The listing builds one solid part. Answer for the finished solid, in the listing's coordinates (mm). A direction names the side the tool comes from. Round coordinates to 2 decimals unless told otherwise and drop trailing zeros. Order: outer loops, then holes, each group sorted by start corner. A loop starts at its lowest first (then second) coordinate and runs counter-clockwise, first axis right, second up. Notation, with made-up numbers: M 30.25,1 L 73.25,1 A13 cw 73.25,16 Z; hole C 62,-29.75 d1. An arc over 180 degrees is marked long. Write item = value, one per line. Start each with the question number.
(1) A cutting plane is placed at A-A, the plane y = 9.5. Determine the outline of the cut face in (x, z).
(2) For a pull along X with two mould halves and no side action, classify faces 1 (the face through (-27.5, 2, 32)), 2 (the face through (-7.615, 1.462, 32.255)), 3 (the face through (-2, 7, 50)), 4 (the face through (-9, 2, 58)) as released by +X, released by -X, zero draft, split by the parting line, or undercut.
(3) Each of these flat-tipped pins is pushed along its axis until it touches: pin 1 (10 mm diameter, centred on y = 7.5, z = 38.5, fed in from +X); pin 2 (6 mm diameter, centred on x = -20, z = 42, fed in from +Y); pin 3 (5 mm diameter, centred on y = 2.5, z = 56, fed in from +X); pin 4 (3 mm diameter, centred on x = -5, z = 44, fed in from +Y). Where does it stop, or does it pass through?
(4) A cutting plane is placed at C-C, the plane z = 8.5. Determine the outline of the cut face in (x, y), and give its area (3 significant figures).
(5) Straight lines are drawn through the part: probe 1 along Y at (x, z) = (0, 28); probe 2 along X at (y, z) = (1.65, 56.5); probe 3 along Y at (x, z) = (-15, 50.5). For each, find the intervals that lie inside material, in ascending order. Write a range as from..to.
(6) Which of the six approach directions +Z, -Z, +X, -X, +Y, -Y give full straight-line access (tool end or side, diameter ignored) to faces 5 (the face through (-2, 7, 15)), 6 (the face through (-18, 2, 65))?
(7) A cutting plane is placed at B-B, the plane x = -21. Determine the outline of the cut face in (y, z).
(8) A cutting plane is placed at D-D, the plane z = 36.5. Determine the outline of the cut face in (x, y), and give its area (3 significant figures).
from build123d import *

# Parameters (mm, degrees)
EXTRUDE_1_DEPTH     = 65
SKETCH_2_R          = 3
CUT_EXTRUDE_1_DEPTH = 65
SKETCH_3_W          = 18
SKETCH_3_H          = 15
CUT_EXTRUDE_2_DEPTH = 25
SKETCH_4_R          = 3
CUT_EXTRUDE_3_DEPTH = 50


with BuildPart() as part:
    # 草图1 → 凸台-拉伸1 (new body)
    with BuildSketch(Plane.XY):
        with BuildLine():
            Line((-27.5, 4.75), (-27.5, 0))
            Line((-27.5, 0), (-9, 0))
            Line((-9, 0), (-6.189701831, 2.966425845))
            ThreePointArc((-6.189701831, 2.966425845), (6.974322263, 15.188482133), (-7.644442426, 4.75))
            Line((-7.644442426, 4.75), (-27.5, 4.75))
        make_face()
    extrude(amount=EXTRUDE_1_DEPTH)

    # 草图2 → 切除-拉伸1 (cut)
    with BuildSketch(Plane(origin=(0, 4.75, 0), x_dir=(1, 0, 0), z_dir=(0, 1, 0))):
        with Locations(Location((-19.5, -8.5, 0), (0, 0, 180))):
            Circle(SKETCH_2_R)
        with Locations(Location((-19.5, -56.5, 0), (0, 0, 270))):
            Circle(SKETCH_2_R)
    extrude(amount=-CUT_EXTRUDE_1_DEPTH, mode=Mode.SUBTRACT)

    # 草图3 → 切除-拉伸2 (cut, symmetric)
    with BuildSketch(Plane(origin=(0, 4.75, 0), x_dir=(1, 0, 0), z_dir=(0, 1, 0))):
        with Locations((0, -7.5)):
            Rectangle(SKETCH_3_W, SKETCH_3_H)
        with Locations((0, -57.5)):
            Rectangle(SKETCH_3_W, SKETCH_3_H)
    extrude(amount=CUT_EXTRUDE_2_DEPTH, both=True, mode=Mode.SUBTRACT)

    # 草图4 → 切除-拉伸3 (cut)
    with BuildSketch(Plane.XY.offset(50)):
        with Locations((0, 9.5)):
            Circle(SKETCH_4_R)
    extrude(amount=-CUT_EXTRUDE_3_DEPTH, mode=Mode.SUBTRACT)


solid = part.part
Reported:
q1.outline = M -9,15 L -3,15 L -3,50 L -9,50 Z; M 3,15 L 9,15 L 9,50 L 3,50 Z
q2.face_1 = released by -X
q2.face_2 = undercut
q2.face_3 = zero draft
q2.face_4 = released by +X
q3.pin_1 = 9
q3.pin_2 = 4.75
q3.pin_3 = -9
q3.pin_4 = 17.79
q4.outline = M -27.5,0 L -22.5,0 L -22.5,4.75 L -27.5,4.75 Z; M -16.5,0 L -9,0 L -9,4.75 L -16.5,4.75 Z
q4.area = 59.4 mm²
q5.probe_1 = 0.5..6.5, 12.5..18.5
q5.probe_2 = -27.5..-22.5, -16.5..-9
q5.probe_3 = 0..4.75
q6.face_5 = -Z, +X, +Y, -Y
q6.face_6 = +Z, +X, -X, +Y, -Y
q7.outline = M 0,0 L 4.75,0 L 4.75,5.9 L 0,5.9 Z; M 0,11.1 L 4.75,11.1 L 4.75,53.9 L 0,53.9 Z; M 0,59.1 L 4.75,59.1 L 4.75,65 L 0,65 Z
q8.outline = M -27.5,0 L -9,0 L -6.19,2.97 A9 ccw long -7.64,4.75 L -27.5,4.75 Z; hole C 0,9.5 d6
q8.area = 322 mm²
